Check sheet for the modelled part. Datum: model origin and axes. Units: mm. A direction names the side the tool comes from. Round coordinates to 2 decimals unless told otherwise and drop trailing zeros. Write item = value, one per line.
from build123d import *

# Parameters (mm, degrees)
HOLE1_D           = 8.4328
CIRPATTERN1_COUNT = 24
EXTRUDE1_DEPTH    = 1.016


with BuildPart() as part:
    # Sketch1 → Revolve1 (revolve)
    with BuildSketch(Plane.XY, mode=Mode.PRIVATE) as revolve1_sk:
        Polygon((255.900825698, 390.490656873), (255.900825698, 381.245056873), (267.330825698, 381.245056873), (267.330825698, 383.886656873), (278.506825698, 383.886656873), (279.268825698, 384.648656873), (279.268825698, 407.889656873), (278.506825698, 408.651656873), (256.409254981, 408.651656873), (255.392825698, 408.649168915), (254.630825698, 407.887153851), (254.630825698, 393.154822015), (255.59724885, 393.157656873), (256.261934313, 393.157656873), (255.291225698, 390.490656873), align=None)
    revolve(revolve1_sk.sketch.rotate(Axis((234.51052404, 282.032656873, 0), (1, 0, 0)), 90), axis=Axis((234.51052404, 282.032656873, 0), (1, 0, 0)))

    # Hole1 (through all)
    with Locations(Plane(origin=(254.630825698, 397.958256873, 0), x_dir=(0, 0, -1), z_dir=(-1, 0, 0))):
        with Locations((0, 0)):
            hole1 = Hole(HOLE1_D / 2)

    # CirPattern1: Hole1 ×24 about axis
    cirpattern1_axis = Axis((0, 282.032656873, 0), (1, 0, 0))
    for i in range(1, CIRPATTERN1_COUNT):
        add(hole1.rotate(cirpattern1_axis, i * 360 / CIRPATTERN1_COUNT), mode=Mode.SUBTRACT)

    # Sketch5 → Extrude1 (cut)
    with BuildSketch(Plane.ZY.offset(-254.630825698)):
        Polygon((17.293788017, 413.392018325), (18.080747375, 413.28841316), (15.154326219, 391.060037623), (13.580407501, 391.267247953), (16.506828658, 413.49562349), align=None)
        Polygon((-19.417001089, 128.464736046), (-20.990919806, 128.671946376), (-15.132677091, 173.169717573), (-13.558758374, 172.962507243), align=None)
    extrude(amount=-EXTRUDE1_DEPTH, mode=Mode.SUBTRACT)


solid = part.part
(1) Material ranges on L1, parallel to Z at x = 263.75, y = 282.5; L2, parallel to Y at x = 260.5, z = -104; L3, parallel to Y at x = 278, z = -110.5, recorded low to high. Write a range as [from, to].
Worked answers:
L1 = [-126.62, -120.12], [-111.74, -99.21], [99.21, 111.74], [120.12, 126.62]
L2 = [209.81, 221.88], [226.26, 337.81], [342.18, 354.26]
L3 = [220.21, 248.08], [255.98, 308.09], [315.99, 343.86]
(2) Sectioned sample at A-A on x = 260.25. Count the separate pieces of the cut face and the enclosed holes in it, then the cut area to 3 significant figures.
Worked answers:
separate_pieces = 1
enclosed_holes = 25
area = 18,100 mm²
(3) Go/stop test with flat-tipped pins: P1, Ø1.5, axis at x = 258, y = 203.5, coming from the -Z side; P2, Ø12, axis at x = 265.5, y = 219, coming from the +Z side; P3, Ø3, axis at x = 261.5, z = 54.5, coming from the -Y side. Record where each tip stops, or that it passes through.
Worked answers:
P1 = -99.91
P2 = 113.05
P3 = 167.04
(4) Access from +Z, -Z, +X, -X, +Y, -Y to the whole of each face (thin tool, end or side, straight path). Record for faces 4 (the cylindrical face through (267.12, 343.55, 98.13)), 5 (the flat face through (267.331, 380, -22)).
Worked answers:
face_4 = +X, -X
face_5 = +X
(5) Release check for a two-part mould opening along X. For faces 1 (the cylindrical face through (267.122, 285.928, -117.541)), 2 (the conical face through (254.752, 295.736, -125.229)), 3 (the conical face through (255.013, 269.943, 110.464)) record: pulls with the +X half, pulls with the -X half, needs draft (parallel to the pull), parting line crosses it, or undercut.
Worked answers:
face_1 = needs draft
face_2 = pulls with the -X half
face_3 = undercut
